Build history of the part. All positions in model axes, mm. A direction names the side the tool comes from. Give positions to 0.01 mm unless a question says otherwise; leave off trailing zeros. Loops run counter-clockwise (first coordinate to the right, second up) from the corner with the lowest first, then second, coordinate; pieces in that order, holes last.
1) Flat gauge pins, fed straight in: P1, Ø4, axis at x = -23.5, y = 30.5, coming from the -Z side; P2, Ø12, axis at x = 23, y = -35.5, coming from the -Z side; P3, Ø4, axis at x = 18.5, z = 198.5, coming from the +Y side. Where does each tip first touch, or does it go through?
2) Two-plate mould, pull along X, no slides. Class faces 1 (the conical face through (14.032, -10.76, 137.274)), 2 (the conical face through (3.92, -17.66, 136.35)), 3 (the flat face through (-17, 27, 234.375)): +X half, -X half, draft (parallel to the pull), parting line (faces both ways), or undercut.
3) Band-saw the part on A-A on x = 21.5. State how many separate pieces and enclosed holes the cut face has, then the cut area to 3 significant figures.
4) Band-saw the part on B-B on z = 119. List the corners of the cut face in (x, y), then the cut area to 3 significant figures.
5) Wall check: line 1 (Z direction, x = -25.5, y = 5); line 2 (Z direction, x = -12, y = 26); line 3 (X direction, y = 9.5, z = 207). Give the ranges that are in metal, low to high.
6) 3-axis set-ups, long thin cutter, end or side, ignore diameter. For faces 4 (the conical face through (-8.203, 2.583, 11.083)), 5 (the conical face through (5.25, 39.98, 206.5)): which of +Z, -Z, +X, -X, +Y, -Y reach the whole face in a straight line?
```python
from build123d import *

# Parameters (mm, degrees)
F2_R = 5
F3_T = -1


with BuildPart() as f1:
    # F0 (on Front) → F1 (revolve)
    with BuildSketch(Plane.XZ):
        Polygon((0, 234.375019135), (-32.5, 234.375019135), (-52.2581860423, 163.971722126), (-47.0857657492, 150.5581885576), (-35.2828800678, 141.1640495062), (-17.2172356397, 136.105671525), (-3.6069871858, 127.5546848774), (-4.0083518252, 13.5655401951), (-36.054097116, 3.551248461), (0, 3.551248461), align=None)
    revolve(axis=Axis((0, 0, 118.963133798), (0, 0, -1)))

    # F2
    f2_edges = [f1.edges().sort_by_distance(p)[0] for p in [
        (4.008352, 0, 13.56554),
        (3.606987, 0, 127.554685),
    ]]
    fillet(f2_edges, radius=F2_R)

    # F3
    f3_openings = [f1.faces().sort_by_distance(p)[0] for p in [
        (0, 0, 234.375019),
    ]]
    offset(amount=F3_T, openings=f3_openings, kind=Kind.INTERSECTION)


solid = f1.part
```
Findings below:
1. P1: stops at z = 142.14
1. P2: stops at z = 141.97
1. P3: stops at y = 39.44
2. face 1: undercut
2. face 2: parting line
2. face 3: draft
3. separate pieces: 2
3. enclosed holes: 1
3. area: 398 mm2
4. outline: circle Ø7.27 at (0, 0); hole circle Ø5.27 at (0, 0)
4. area: 19.7 mm2
5. line 1: z = 3.55 to 4.55, 5.65 to 6.7, 138.56 to 139.6
5. line 2: z = 3.55 to 4.55, 4.82 to 5.87, 139.3 to 140.34
5. line 3: x = -39.04 to -37.97, 37.97 to 39.04
6. face 4: none
6. face 5: +Z
